from build123d import *

# Parameters (mm, degrees)
SKETCH1_R               = 1
BOSS_EXTRUDE1_DEPTH     = 12
SKETCH2_R               = 3.3
CUT_EXTRUDE1_DEPTH      = 2.5
CUT_EXTRUDE1_DEPTH_BACK = 2.5
FILLET1_R               = 1
FILLET2_R               = 1
FILLET3_R               = 1
FILLET4_R               = 0.5
FILLET5_R               = 0.25


with BuildPart() as part:
    # Sketch1 → Boss-Extrude1 (new body)
    with BuildSketch(Plane.XY):
        with BuildLine():
            Line((0, 0), (21.817354946, 0))
            ThreePointArc((21.817354946, 0), (23.938675289, 5.121320344), (18.817354946, 3))
            Line((18.817354946, 3), (4, 5.97347684))
            Line((4, 5.97347684), (4, 23.200108131))
            Line((4, 23.200108131), (6.297593783, 30.327226275))
            ThreePointArc((6.297593783, 30.327226275), (11.237097985, 31.191049803), (8.483562347, 35.381865278))
            Line((8.483562347, 35.381865278), (0, 35.381865278))
            Line((0, 35.381865278), (0, 0))
        make_face()
        with Locations((8.483562347, 32.381865278)):
            Circle(SKETCH1_R, mode=Mode.SUBTRACT)
        with Locations((21.817354946, 3)):
            Circle(SKETCH1_R, mode=Mode.SUBTRACT)
        Polygon((5.180971974, 33.381865278), (2, 33.381865278), (2, 23.514514817), align=None, mode=Mode.SUBTRACT)
        Polygon((2, 2), (2, 4.334954297), (13.63548548, 2), align=None, mode=Mode.SUBTRACT)
    extrude(amount=BOSS_EXTRUDE1_DEPTH)

    # Sketch2 → Cut-Extrude1 (cut, two sides)
    with BuildSketch(Plane.XY.offset(6)) as cut_extrude1_sk:
        with Locations((8.483562347, 32.381865278)):
            Circle(SKETCH2_R)
        with Locations((21.817354946, 3)):
            Circle(SKETCH2_R)
    extrude(amount=CUT_EXTRUDE1_DEPTH, mode=Mode.SUBTRACT)
    extrude(cut_extrude1_sk.sketch, amount=-CUT_EXTRUDE1_DEPTH_BACK, mode=Mode.SUBTRACT)

    # Fillet1
    fillet1_edges = [part.edges().sort_by_distance(p)[0] for p in [
        (0, 35.381865278, 6),
        (0, 0, 6),
    ]]
    fillet(fillet1_edges, radius=FILLET1_R)

    # Fillet2
    fillet2_edges = [part.edges().sort_by_distance(p)[0] for p in [
        (4, 23.200108131, 6),
        (4, 5.97347684, 6),
    ]]
    fillet(fillet2_edges, radius=FILLET2_R)

    # Fillet3
    fillet3_edges = [part.edges().sort_by_distance(p)[0] for p in [
        (7.108789639, 35.381865278, 6),
        (20.442582237, 0, 6),
    ]]
    fillet(fillet3_edges, radius=FILLET3_R)

    # Fillet4
    fillet4_edges = [part.edges().sort_by_distance(p)[0] for p in [
        (2, 2, 6),
        (2, 4.334954297, 6),
        (2, 23.514514817, 6),
        (5.180971974, 33.381865278, 6),
        (2, 33.381865278, 6),
    ]]
    fillet(fillet4_edges, radius=FILLET4_R)

    # Fillet5
    fillet5_edges = [part.edges().sort_by_distance(p)[0] for p in [
        (13.63548548, 2, 6),
    ]]
    fillet(fillet5_edges, radius=FILLET5_R)


solid = part.part
The listing builds one solid part. Answer for the finished solid, in the listing's coordinates (mm). A direction names the side the tool comes from. Coordinates: 2 decimals unless noted, no trailing zeros. Loops run counter-clockwise (first coordinate to the right, second up) from the corner with the lowest first, then second, coordinate; pieces in that order, holes last.
1) Flat-ended cylindrical pins translate along their axes: pin 1 Ø6 at (x, y) = (9, 23) entering from -Z; pin 2 Ø1.9 at (y, z) = (31, 7.5) entering from +X. Find the tip coordinate at first contact, or state that the pin passes through.
2) Find section C-C on x = 20. Write down the section's boundary in (y, z), then the cut area to 3 significant figures.
3) Find section D-D on z = 2. Write down the section's boundary in (x, y), then the cut area to 3 significant figures.
4) Find the intervals of material crossed by L1, parallel to Y at x = 2.25, z = 6.5; L2, parallel to Y at x = 9.25, z = 10; L3, parallel to Y at x = 9.75, z = 2.25, in increasing order.
5) Find section A-A on x = 10.25. Write down the section's boundary in (y, z), then the cut area to 3 significant figures.
6) A tool of negligible diameter and unlimited length cuts with its end or side. For faces 1 (the face through (11, 0, 6)), 2 (the face through (7, 2, 6)), 3 (the face through (4, 15, 6)), from which of +Z, -Z, +X, -X, +Y, -Y can it reach the whole face along a straight path? Write none if from no direction.
7) Find section B-B on z = 7.25. Write down the section's boundary in (x, y).
8) Determine the mould class of faces 4 (the face through (5.525, 34.911, 5.965)), 5 (the face through (0.301, 35.097, 6.084)), 6 (the face through (24.01, 5.05, 10.23)) for opening direction X: pulls with the +X half, pulls with the -X half, needs draft (parallel to the pull), parting line crosses it, or undercut.
Values:
1. pin 1: passes through
1. pin 2: stops at x = 6.15
2. outline: (0, 0) - (5.39, 0) - (5.39, 3.5) - (0, 3.5) - close; (0, 8.5) - (5.39, 8.5) - (5.39, 12) - (0, 12) - close
2. area: 37.7 mm2
3. outline: (0, 1) arc R1 ccw to (1, 0) - (21.82, 0) arc R3 ccw (long way) to (18.82, 3) - (4.8, 5.81) arc R1 cw to (4, 6.79) - (4, 23.04) arc R1 cw to (4.05, 23.35) - (6.3, 30.33) arc R3 ccw (long way) to (8.48, 35.38) - (1, 35.38) arc R1 ccw to (0, 34.38) - close; hole (2, 2.5) arc R0.5 ccw to (2.5, 2) - (11.12, 2) arc R0.25 ccw to (11.17, 2.5) - (2.6, 4.21) arc R0.5 ccw to (2, 3.72) - close; hole (2, 26.7) arc R0.5 ccw to (2.98, 26.54) - (4.97, 32.73) arc R0.5 ccw to (4.49, 33.38) - (2.5, 33.38) arc R0.5 ccw to (2, 32.88) - close; hole circle Ø2 at (8.48, 32.38); hole circle Ø2 at (21.82, 3)
3. area: 251 mm2
4. L1: y = 0 to 2.07, 4.16 to 26.26, 33.31 to 35.38
4. L2: y = 0 to 2, 2.88 to 4.92, 29.48 to 31.74, 33.02 to 35.28
4. L3: y = 0 to 2, 2.78 to 4.82, 29.66 to 35.1
5. outline: (0, 0) - (2, 0) - (2, 12) - (0, 12) - close; (2.68, 0) - (4.72, 0) - (4.72, 12) - (2.68, 12) - close; (29.96, 0) - (34.81, 0) - (34.81, 3.5) - (29.96, 3.5) - close; (29.96, 8.5) - (34.81, 8.5) - (34.81, 12) - (29.96, 12) - close
5. area: 82.4 mm2
6. face 1: +Z, -Z, +X, -X, -Y
6. face 2: +Z, -Z
6. face 3: +Z, -Z, +X
7. outline: (0, 1) arc R1 ccw to (1, 0) - (18.01, 0) arc R1 ccw to (18.9, 1.47) arc R3.3 cw to (18.52, 3.06) - (4.8, 5.81) arc R1 cw to (4, 6.79) - (4, 23.04) arc R1 cw to (4.05, 23.35) - (6.19, 30.01) arc R3.3 cw to (5.56, 33.92) arc R1 ccw to (4.68, 35.38) - (1, 35.38) arc R1 ccw to (0, 34.38) - close; hole (2, 2.5) arc R0.5 ccw to (2.5, 2) - (11.12, 2) arc R0.25 ccw to (11.17, 2.5) - (2.6, 4.21) arc R0.5 ccw to (2, 3.72) - close; hole (2, 26.7) arc R0.5 ccw to (2.98, 26.54) - (4.97, 32.73) arc R0.5 ccw to (4.49, 33.38) - (2.5, 33.38) arc R0.5 ccw to (2, 32.88) - close
8. face 4: pulls with the +X half
8. face 5: pulls with the -X half
8. face 6: undercut
